Geometry: final body of the model. Coordinates: model frame, mm. Face numbers are marked on the shaded views. A direction names the side the tool comes from. Give positions to 0.01 mm unless a question says otherwise; leave off trailing zeros. Order: outer loops, then holes, each group sorted by start corner. A loop starts at its lowest first (then second) coordinate and runs counter-clockwise, first axis right, second up. Notation, with made-up numbers: (-20, 73.5) - (-16, 73.5) arc R24 ccw to (-16, 98.5) - close; hole circle Ø4 at (47, 48.5). An arc over 180 degrees is marked (long way). Put each result on its own line as item: value. Start each with the question number.
1. First-contact query: P1, Ø4, axis at x = 14, z = 7, coming from the +Y side; P2, Ø3, axis at y = 14.5, z = 9.5, coming from the -X side; P3, Ø5, axis at y = 17, z = 1.5, coming from the +X side. Flat tips, straight axial feed; report the tip coordinate or a pass-through.
2. Section B-B on y = 1.75. Return the cut outline in (x, z).
3. Section D-D on y = 12.7. Return the cut outline in (x, z).
4. Section C-C on z = 7.25. Return the cut outline in (x, y).
5. Set-up query: the marked faces 5 and 6. Return all of +Z, -Z, +X, -X, +Y, -Y with unobstructed straight access to the full face (end or side cutting, diameter ignored); none if empty.
6. Ray query, line 1 along Z through (x, y) = (0.7, 12.7); line 2 along Z through (x, y) = (12.7, 0.7); line 3 along X through (y, z) = (2, 6.35). Return the intervals inside material, ascending. Write a range as from..to.
7. Mould query, pull axis Y, two halves, no side actions, for the marked faces 1, 2, 3 and 4. Classes: pulls with the +Y half, pulls with the -Y half, needs draft (parallel to the pull), parting line crosses it, or undercut.
8. Section A-A on x = 12.7. Return the cut outline in (y, z), plus the area to 3 significant figures.
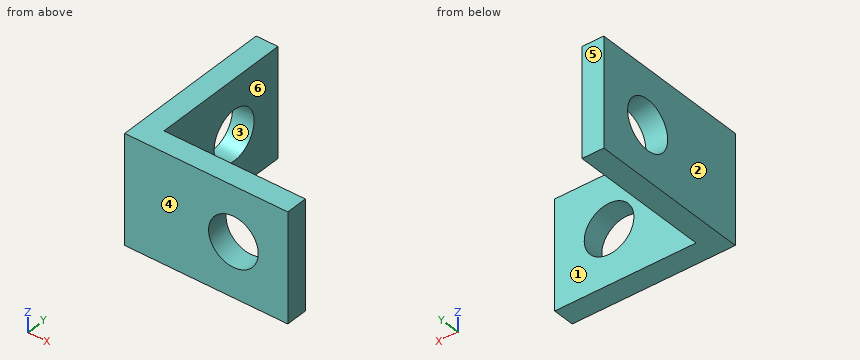
from build123d import *

# Parameters (mm, degrees)
BOSS_EXTRUDE1_DEPTH = 12.7
SKETCH2_R           = 2.9
CUT_EXTRUDE1_DEPTH  = 12.7
SKETCH3_R           = 2.9
CUT_EXTRUDE3_DEPTH  = 12.7


with BuildPart() as part:
    # Sketch1 → Boss-Extrude1 (new body)
    with BuildSketch(Plane.XY):
        Polygon((0, 0), (0, 19.05), (2.54, 19.05), (2.54, 2.54), (19.05, 2.54), (19.05, 0), align=None)
    extrude(amount=BOSS_EXTRUDE1_DEPTH)

    # Sketch2 → Cut-Extrude1 (cut)
    with BuildSketch(Plane(origin=(0, 0, 0), x_dir=(0, 0, -1), z_dir=(1, 0, 0))):
        with Locations(Location((-6.299909987, 12.7, 0), (0, 0, 180))):
            Circle(SKETCH2_R)
    extrude(amount=CUT_EXTRUDE1_DEPTH, mode=Mode.SUBTRACT)

    # Sketch3 → Cut-Extrude3 (cut)
    with BuildSketch(Plane(origin=(0, 0, 0), x_dir=(1, 0, 0), z_dir=(0, 1, 0))):
        with Locations(Location((12.7, -6.35, 0), (0, 0, 90))):
            Circle(SKETCH3_R)
    extrude(amount=CUT_EXTRUDE3_DEPTH, mode=Mode.SUBTRACT)


solid = part.part
Resolved:
1. P1: y = 2.54
1. P2: x = 0
1. P3: x = 2.54
2. outline: (0, 0) - (19.05, 0) - (19.05, 12.7) - (0, 12.7) - close; hole circle Ø5.8 at (12.7, 6.35)
3. outline: (0, 0) - (2.54, 0) - (2.54, 3.4) - (0, 3.4) - close; (0, 9.2) - (2.54, 9.2) - (2.54, 12.7) - (0, 12.7) - close
4. outline: (0, 0) - (9.94, 0) - (9.94, 2.54) - (2.54, 2.54) - (2.54, 9.96) - (0, 9.96) - close; (0, 15.44) - (2.54, 15.44) - (2.54, 19.05) - (0, 19.05) - close; (15.46, 0) - (19.05, 0) - (19.05, 2.54) - (15.46, 2.54) - close
5. face 5: +Z, -Z, +X, -X, +Y
5. face 6: +Z, -Z, +X, +Y
6. line 1: 0..3.4, 9.2..12.7
6. line 2: 0..3.45, 9.25..12.7
6. line 3: 0..9.8, 15.6..19.05
7. face 1: pulls with the +Y half
7. face 2: needs draft
7. face 3: undercut
7. face 4: pulls with the -Y half
8. outline: (0, 0) - (2.54, 0) - (2.54, 3.45) - (0, 3.45) - close; (0, 9.25) - (2.54, 9.25) - (2.54, 12.7) - (0, 12.7) - close
8. area: 17.5 mm^2
